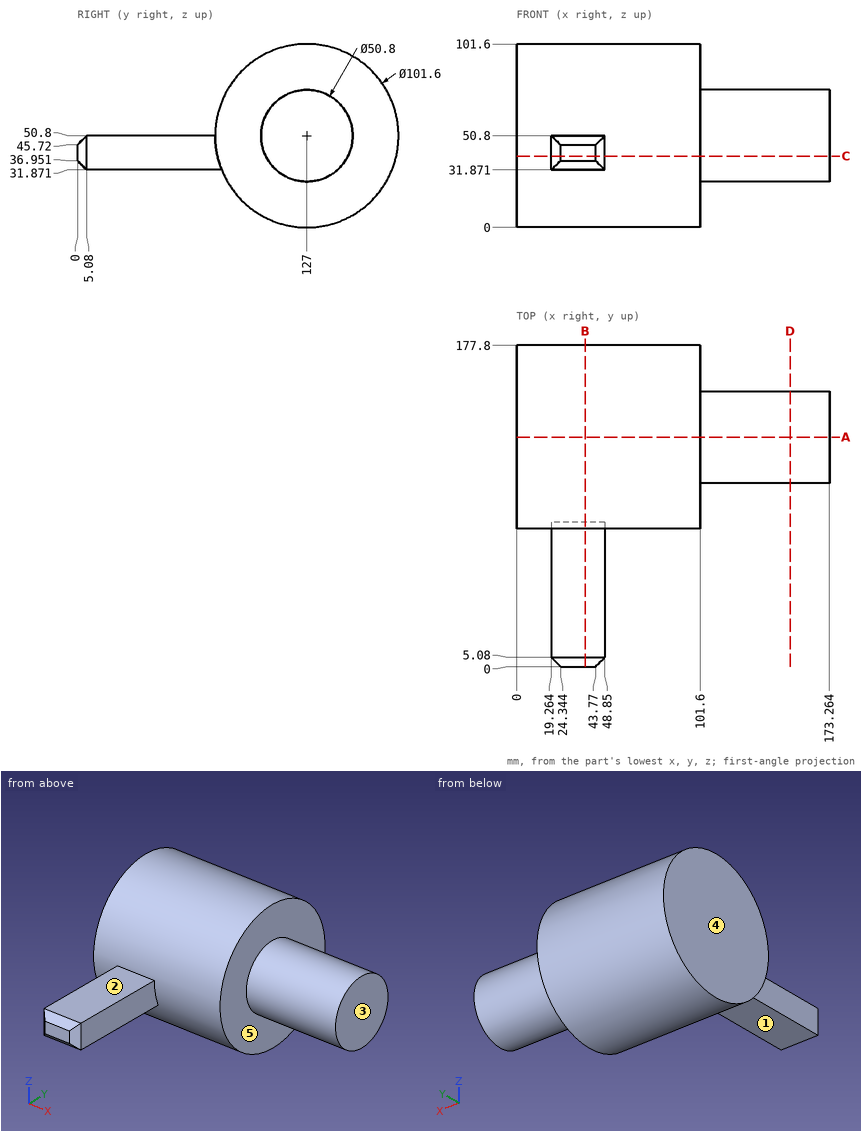
Could you check a few things on this drawing? It's one solid part, dimensions in mm from its lowest x, y, z. A direction names the side the tool comes from. Give positions to 0.01 mm unless a question says otherwise; leave off trailing zeros. Order: outer loops, then holes, each group sorted by start corner. A loop starts at its lowest first (then second) coordinate and runs counter-clockwise, first axis right, second up.
1. I need wall thicknesses on L1, parallel to X at y = 154, z = 63; L2, parallel to X at y = 30, z = 46; L3, parallel to Z at x = 27.5, y = 48. Which ranges of each line are inside material? Lowest first, please.
Answers below:
L1: x = 0 to 101.6
L2: x = 19.26 to 48.85
L3: z = 31.87 to 50.8
2. Suppose I cut it at B-B (x = 38). Write out the boundary of the cut face in (y, z), plus the area to 3 significant figures.
Answers below:
outline: (0, 36.95) - (5.08, 31.87) - (79.86, 31.87) arc R50.8 ccw (long way) to (76.2, 50.8) - (5.08, 50.8) - (0, 45.72) - close
area: 9,550 mm2
3. Suppose I cut it at C-C (z = 39.5). Write out the boundary of the cut face in (x, y), plus the area to 3 significant figures.
Answers below:
outline: (0, 77.47) - (19.26, 77.47) - (19.26, 5.08) - (24.34, 0) - (43.77, 0) - (48.85, 5.08) - (48.85, 77.47) - (101.6, 77.47) - (101.6, 104.25) - (173.26, 104.25) - (173.26, 149.75) - (101.6, 149.75) - (101.6, 176.53) - (0, 176.53) - close
area: 15,600 mm2
4. For pin 1 (1.5 mm diameter, centred on x = 71.5, z = 52, fed in from +Y); pin 2 (6 mm diameter, centred on x = 136, z = 42, fed in from -Y); pin 3 (3 mm diameter, centred on x = 66, z = 62.5, fed in from -Y) (1 decimal), each with a flat end and sliding along its axis, tell me the tip position at first contact or that it passes through.
Answers below:
pin 1: stops at y = 177.8
pin 2: stops at y = 102.27
pin 3: stops at y = 77.2
5. Suppose I cut it at D-D (x = 151.5). Write out the boundary of the cut face in (y, z).
Answers below:
outline: circle Ø50.8 at (127, 50.8)
6. Which directions (+Z, -Z, +X, -X, +Y, -Y) give clear straight access to the entire face, cutting with the end or side of a thin tool? Please do the marked faces 1, 2, 3, 4 and 5.
Answers below:
face 1: -Z, +X, -X, -Y
face 2: +Z, +X, -X, -Y
face 3: +Z, -Z, +X, +Y, -Y
face 4: +Z, -Z, -X, +Y, -Y
face 5: +X
7. Suppose I cut it at A-A (y = 127). Write out the boundary of the cut face in (x, z).
Answers below:
outline: (0, 0) - (101.6, 0) - (101.6, 25.4) - (173.26, 25.4) - (173.26, 76.2) - (101.6, 76.2) - (101.6, 101.6) - (0, 101.6) - close
